Autodesk Inventor part; units mm, degrees
ref_plane "YZ Plane" through (0, 0, 0) normal (1, 0, 0) x (0, 1, 0)
ref_plane "XZ Plane" through (0, 0, 0) normal (0, 1, 0) x (-1, 0, 0)
ref_plane "XY Plane" through (0, 0, 0) normal (0, 0, 1) x (1, 0, 0)
sketch "スケッチ1" plane through (0, 0, 0) normal (0, 1, 0) x (-1, 0, 0)
  circle A0 centre (0, 0) radius 6
  dimension "d0" = 12
extrude "押し出し1" add sketch "スケッチ1" along normal blind 2.2
sketch "スケッチ2" plane through (0, 0, 0) normal (0, -1, 0) x (1, 0, 0)
  circle A0 centre (0, 0) radius 6
  line L0 (-5.9161, 1) -> (-8.4161, 1)
  line L1 (-8.4161, 1) -> (-8.4161, -1)
  line L2 (-8.4161, -1) -> (-5.9161, -1)
  line L3 (-5.9161, -1) -> (-5.9161, 1)
  circle A1 centre (0, 0) radius 6
  dimension "d3" = 2
  dimension "d4" = 2.5
extrude "押し出し2" add sketch "スケッチ2" against normal blind 0.5 contours L3 A0 | A0 L2 L1 L0 picked at (-5.941, 0.1116)
properties part number "motor"
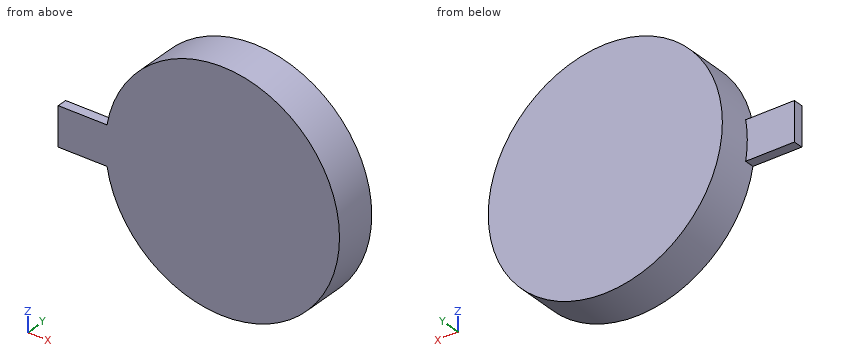
Verification items for the finished model (mm, model axes). Round coordinates to 2 decimals unless told otherwise and drop trailing zeros. Order: outer loops, then holes, each group sorted by start corner. A loop starts at its lowest first (then second) coordinate and runs counter-clockwise, first axis right, second up. Notation, with made-up numbers: (22, -33) -> (62, -33) arc R7 ccw to (62, -26) -> close; hole circle Ø9 at (-25.75, 24.5). An arc over 180 degrees is marked (long way). Put each result on its own line as item: value.
1) Section check B-B (y = 1.2). Record the cut outline in (x, z).
Final values:
outline: circle Ø12 at (0, 0)
2) Material ranges on line 1 (Z direction, x = -7.5, y = 0.3); line 2 (X direction, y = 0.3, z = 5); line 3 (X direction, y = 1.05, z = -3.75), recorded low to high.
Final values:
line 1: z = -1 to 1
line 2: x = -3.32 to 3.32
line 3: x = -4.68 to 4.68
3) Section check D-D (z = -4). Record the cut outline in (x, y), then the cut area to 3 significant figures.
Final values:
outline: (-4.47, 0) -> (4.47, 0) -> (4.47, 2.2) -> (-4.47, 2.2) -> close
area: 19.7 mm^2
4) Section check C-C (x = -4). Record the cut outline in (y, z).
Final values:
outline: (0, -4.47) -> (2.2, -4.47) -> (2.2, 4.47) -> (0, 4.47) -> close
5) Section check A-A (z = 0). Record the cut outline in (x, y), then the cut area to 3 significant figures.
Final values:
outline: (-8.42, 0) -> (6, 0) -> (6, 2.2) -> (-6, 2.2) -> (-6, 0.5) -> (-8.42, 0.5) -> close
area: 27.6 mm^2
